Autodesk Inventor part; units mm, degrees
ref_plane "YZ Plane" through (0, 0, 0) normal (1, 0, 0) x (0, 1, 0)
ref_plane "XZ Plane" through (0, 0, 0) normal (0, 1, 0) x (-1, 0, 0)
ref_plane "XY Plane" through (0, 0, 0) normal (0, 0, 1) x (1, 0, 0)
sketch "Sketch1" plane through (0, 0, 0) normal (0, 0, 1) x (1, 0, 0)
  circle A0 centre (0, 0) radius 5
  dimension "d0" = 10
extrude "Extrusion1" add sketch "Sketch1" along normal blind 30 draft -3
sketch "Sketch2" plane through (0, 0, 30) normal (0, 0, 1) x (1, 0, 0)
  circle A0 centre (0, 0) radius 2.8754
extrude "Extrusion2" add sketch "Sketch2" along normal blind 5
fillet "Fillet1" radius 2 1 edges at (-2.8754, 0, 35)
sketch "Sketch4" plane through (0, 0, 0) normal (0, 1, 0) x (-1, 0, 0)
  circle A0 centre (0, 31.4792) radius 1.25
  point P0 (0, 0)
  dimension "d8" = 2.5
extrude "Extrusion4" cut sketch "Sketch4" along normal mid plane 10
sketch "Sketch5" plane through (0, 0, 35) normal (0, 0, 1) x (1, 0, 0)
  circle A0 centre (0, 0) radius 5
  line L0 (-4.6538, 1.8283) -> (4.6538, 1.8283)
  line L1 (4.6538, -1.8283) -> (-4.6538, -1.8283)
  arc A1 (-4.6538, 1.8283) -> (-4.6538, -1.8283) centre (0, 0) ccw
  arc A2 (4.6538, -1.8283) -> (4.6538, 1.8283) centre (0, 0) ccw
extrude "Extrusion5" cut sketch "Sketch5" against normal blind 10 contours A0 L1 L0
properties part number "arms"
Geometry: final body of the model. Coordinates: model frame, mm. A direction names the side the tool comes from. Round coordinates to 2 decimals unless told otherwise and drop trailing zeros. Order: outer loops, then holes, each group sorted by start corner. A loop starts at its lowest first (then second) coordinate and runs counter-clockwise, first axis right, second up. Notation, with made-up numbers: (37, 88.5) - (73, 88.5) arc R26 cw to (73, 110.5) - close; hole circle Ø4 at (45, 16.25). An arc over 180 degrees is marked (long way). Write each question's results on one line, items separated by ' | '.
Item 1: Section C-C, the plane y = 0. Return the cut outline in (x, z), and give its area (3 significant figures).
Completed:
outline: (-5, 0) - (5, 0) - (3.69, 25) - (-3.69, 25) - close | area: 217 mm^2
Item 2: Section B-B, the plane x = 0. State how many separate pieces and enclosed holes the cut face has, and give its area (3 significant figures).
Completed:
separate pieces: 3 | enclosed holes: 0 | area: 238 mm^2
Item 3: Section A-A, the plane z = 32. Return the cut outline in (x, y).
Completed:
outline: (-2.22, -1.83) arc R2.88 ccw to (-1.14, -2.64) - (-1.14, -1.83) - close; (-2.22, 1.83) - (-1.14, 1.83) - (-1.14, 2.64) arc R2.88 ccw to start; (1.14, -2.64) arc R2.88 ccw to (2.22, -1.83) - (1.14, -1.83) - close; (1.14, 1.83) - (2.22, 1.83) arc R2.88 ccw to (1.14, 2.64) - close
Item 4: Mould query, pull axis Z, two halves, no side actions, for faces 4 (the flat face through (0, 0, 0)), 5 (the cylindrical face through (0.992, -2.345, 30.719)), 6 (the flat face through (0, -3.1, 30)). Classes: pulls with the +Z half, pulls with the -Z half, needs draft (parallel to the pull), parting line crosses it, or undercut.
Completed:
face 4: pulls with the -Z half | face 5: undercut | face 6: pulls with the +Z half
Item 5: Reachability of faces 1 (the flat face through (0, 3.2, 30)), 2 (the cylindrical face through (0.99, 2.34, 32.24)), 3 (the flat face through (0, -1.828, 29)) from +Z, -Z, +X, -X, +Y, -Y: full face, straight path, thin tool, end or side. Return the list, or none.
Completed:
face 1: +Z, +Y | face 2: +Y, -Y | face 3: +Z, +X, -X
Item 6: Material intervals for line 1 along X through (y, z) = (-1.75, 22); line 2 along Z through (x, y) = (0, 2.15); line 3 along Z through (x, y) = (0, -2.6), sorted ascending. Write a range as [from, to].
Completed:
line 1: [-3.43, 3.43] | line 2: [0, 30.23], [32.73, 34.54] | line 3: [0, 30.23], [32.73, 34.01]
Item 7: Section D-D, the plane z = 6. Return the cut outline in (x, y).
Completed:
outline: circle Ø9.37 at (0, 0)
Item 8: First-contact query: pin 1 Ø2 at (x, y) = (-1, -4) entering from +Z; pin 2 Ø3 at (x, z) = (-1, 32) entering from +Y; pin 3 Ø4 at (x, z) = (-0.5, 24) entering from -Y; pin 4 Ø1 at (x, y) = (4, -2) entering from -Z. Flat tips, straight axial feed; report the tip coordinate or a pass-through.
Completed:
pin 1: z = 30 | pin 2: y = 2.88 | pin 3: y = -3.84 | pin 4: z = 0
